Autodesk Inventor part; units mm, degrees
ref_plane "YZ Plane" through (0, 0, 0) normal (1, 0, 0) x (0, 1, 0)
ref_plane "XZ Plane" through (0, 0, 0) normal (0, 1, 0) x (-1, 0, 0)
ref_plane "XY Plane" through (0, 0, 0) normal (0, 0, 1) x (1, 0, 0)
sketch "Sketch1" plane through (0, 0, 0) normal (1, 0, 0) x (0, 1, 0)
  line L0 (0, 0) -> (10, 0)
  line L1 (10, 0) -> (10, -10)
  line L2 (10, -10) -> (0, -10)
  line L3 (0, -10) -> (0, 0)
  dimension "d0" = 10
  dimension "d1" = 10
extrude "Extrusion1" add sketch "Sketch1" along normal blind 10
sketch "Sketch4" plane through (0, 0, 0) normal (0, 0, 1) x (1, 0, 0)
  line L0 (1.8731, 7.9408) -> (4.4271, 7.9408) construction
  line L1 (4.4271, 7.9408) -> (4.4271, 4.8928) construction
  line L2 (4.4271, 4.8928) -> (1.8731, 4.8928) construction
  line L3 (1.8731, 4.8928) -> (1.8731, 7.9408) construction
  spline S0 degree 2 poles (7.0108, 6.9784) (6.7321, 6.9784) (6.1484, 7.0258) knots 0 0 0 1 1 1
  spline S1 degree 2 poles (6.1484, 7.0258) (5.5857, 7.0678) (5.2912, 7.0626) knots 0 0 0 1 1 1
  line L4 (5.2912, 7.0626) -> (5.023, 7.0626)
  spline S2 degree 2 poles (5.023, 7.0626) (5.0336, 6.542) (5.1229, 5.3693) knots 0 0 0 1 1 1
  spline S3 degree 2 poles (5.1229, 5.3693) (5.2071, 4.2808) (5.2071, 3.676) knots 0 0 0 1 1 1
  spline S4 degree 2 poles (5.2071, 3.676) (5.2071, 3.5445) (5.2597, 3.0082) (5.2597, 2.8714) knots 0 0 0 1 2 2 2
  spline S5 degree 2 poles (5.2597, 2.8714) (5.2597, 2.619) (5.1755, 2.4297) knots 0 0 0 1 1 1
  spline S6 degree 2 poles (5.1755, 2.4297) (5.0704, 2.1826) (4.8495, 2.1826) knots 0 0 0 1 1 1
  spline S7 degree 2 poles (4.8495, 2.1826) (4.697, 2.1826) (4.4551, 2.3929) (4.4551, 2.5612) knots 0 0 0 1 2 2 2
  spline S8 degree 2 poles (4.4551, 2.5612) (4.4551, 2.619) (4.4919, 2.8452) (4.4919, 2.8977) knots 0 0 0 1 2 2 2
  spline S9 degree 2 poles (4.4919, 2.8977) (4.4919, 3.087) (4.4446, 3.8233) (4.4446, 4.0126) knots 0 0 0 1 2 2 2
  spline S10 degree 2 poles (4.4446, 4.0126) (4.4446, 4.5542) (4.3552, 5.5323) knots 0 0 0 1 1 1
  spline S11 degree 2 poles (4.3552, 5.5323) (4.2658, 6.584) (4.2553, 7.0468) knots 0 0 0 1 1 1
  line L5 (4.2553, 7.0468) -> (3.9135, 7.0415)
  spline S12 degree 2 poles (3.9135, 7.0415) (3.0879, 7.0415) (2.6146, 7.1625) knots 0 0 0 1 1 1
  spline S13 degree 2 poles (2.6146, 7.1625) (2.3096, 7.2414) (2.3096, 7.5358) knots 0 0 0 1 1 1
  spline S14 degree 2 poles (2.3096, 7.5358) (2.3096, 7.6936) (2.4095, 7.8093) knots 0 0 0 1 1 1
  spline S15 degree 2 poles (2.4095, 7.8093) (2.5199, 7.9408) (2.6987, 7.9302) knots 0 0 0 1 1 1
  spline S16 degree 2 poles (2.6987, 7.9302) (2.8302, 7.925) (3.3035, 7.8619) knots 0 0 0 1 1 1
  spline S17 degree 2 poles (3.3035, 7.8619) (3.6768, 7.8146) (3.9135, 7.8146) knots 0 0 0 1 1 1
  spline S18 degree 2 poles (3.9135, 7.8146) (4.1396, 7.8146) (5.0598, 7.8356) (5.286, 7.8356) knots 0 0 0 1 2 2 2
  spline S19 degree 2 poles (5.286, 7.8356) (5.5752, 7.8356) (6.7163, 7.7514) (7.0108, 7.7514) knots 0 0 0 1 2 2 2
  spline S20 degree 2 poles (7.0108, 7.7514) (7.1686, 7.7514) (7.3894, 7.5306) (7.3894, 7.3623) knots 0 0 0 1 2 2 2
  spline S21 degree 2 poles (7.3894, 7.3623) (7.3894, 7.2045) (7.1686, 6.9784) (7.0108, 6.9784) knots 0 0 0 1 2 2 2
  point P0 (0, 0)
extrude "Extrusion4" cut sketch "Sketch4" against normal blind 2
sketch "Sketch7" plane through (0, 0, 0) normal (-1, 0, 0) x (0, 0, 1)
  line L0 (-3.1, 3.1) -> (-6.2, 3.1)
  line L1 (-6.2, 3.1) -> (-6.2, 6.2)
  line L2 (-6.2, 6.2) -> (-3.1, 6.2)
  line L3 (-3.1, 6.2) -> (-3.1, 3.1)
  point P0 (0, 0)
  dimension "d16" = 3.1
  dimension "d17" = 3.1
extrude "Extrusion6" cut sketch "Sketch7" against normal blind 5
properties part number "Thymine"
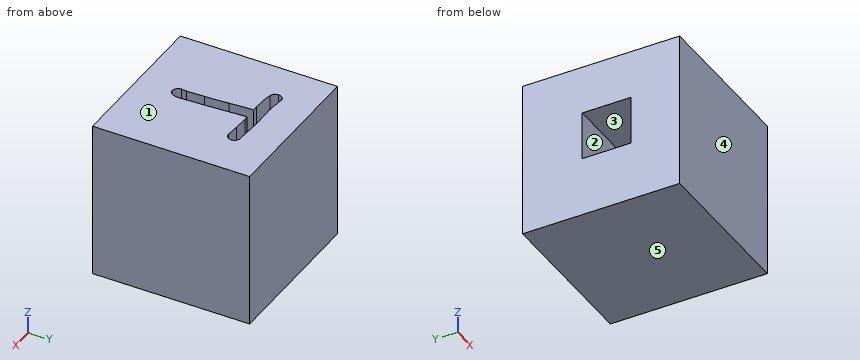
Could you check a few things on this model? Use its own coordinates, in mm. Face numbers are marked on the shaded views. A direction names the side the tool comes from. Coordinates: 2 decimals unless noted, no trailing zeros. Write each loop counter-clockwise with the first axis right and the second up, starting at its lowest first coordinate (ties: lowest second). Pieces come first, ordered by that corner, then holes. Notation, with made-up numbers: (-24, 51) -> (22, 51) arc R28 ccw to (22, 80) -> close; hole circle Ø3 at (-13, 65.5). An arc over 180 degrees is marked (long way). Return JSON: item names as keys, results as strings.
(1) I need wall thicknesses on L1, parallel to Z at x = 3.5, y = 4.25; L2, parallel to Y at x = 1, z = -5.5; L3, parallel to Z at x = 5, y = 7.5. Which ranges of each line are inside material? Lowest first, please.
Numbers:
{"L1": "z = -10 to -6.2, -3.1 to 0", "L2": "y = 0 to 3.1, 6.2 to 10", "L3": "z = -10 to -2"}
(2) Which directions (+Z, -Z, +X, -X, +Y, -Y) give clear straight access to the entire face, cutting with the end or side of a thin tool? Please do the marked faces 1 and 2.
Numbers:
{"face 1": "+Z, +X, -X, +Y, -Y", "face 2": "-X"}
(3) We'd pull the mould along Z, two halves only. Please class the marked faces 3, 4 and 5: +Z half, -Z half, draft (parallel to the pull), parting line (faces both ways), or undercut.
Numbers:
{"face 3": "undercut", "face 4": "draft", "face 5": "-Z half"}
(4) I'm going to push a flat-ended pin straight in: pin 1 (2 mm diameter, centred on y = 1.5, z = -1, fed in from -X). Where does the tip first touch, or does it pass through?
Numbers:
{"pin 1": "stops at x = 0"}
(5) Imagine slicing it at B-B, the plane x = 2. Please give me the cut outline in (y, z).
Numbers:
{"outline": "(0, -10) -> (10, -10) -> (10, 0) -> (0, 0) -> close; hole (3.1, -6.2) -> (6.2, -6.2) -> (6.2, -3.1) -> (3.1, -3.1) -> close"}
(6) Imagine slicing it at A-A, the plane z = -6. Please give me the cut outline in (x, y), then the cut area to 3 significant figures.
Numbers:
{"outline": "(0, 0) -> (10, 0) -> (10, 10) -> (0, 10) -> (0, 6.2) -> (5, 6.2) -> (5, 3.1) -> (0, 3.1) -> close", "area": "84.5 mm2"}
